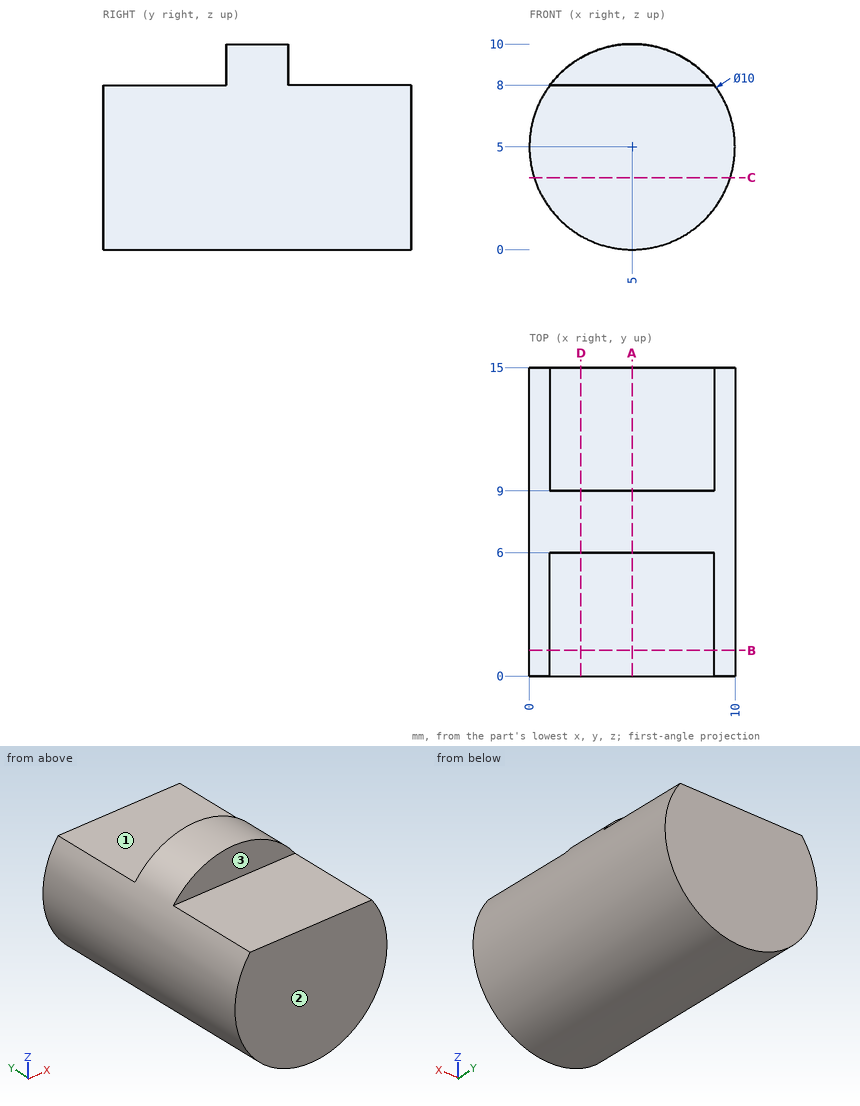
Source: three-view drawing plus pictorial views. Frame: mm from the lowest corner of the part. A direction names the side the tool comes from. Coordinates: 2 decimals unless noted, no trailing zeros. Loops run counter-clockwise (first coordinate to the right, second up) from the corner with the lowest first, then second, coordinate; pieces in that order, holes last. Notation, with made-up numbers: M 35,-23.5 L 64,-23.5 A34 ccw 64,8.5 Z; hole C 52,45 d8. An arc over 180 degrees is marked long. Use CSV: the item, a comma, the result in double quotes.
(1) Reachability of the marked faces 1, 2 and 3 from +Z, -Z, +X, -X, +Y, -Y: full face, straight path, thin tool, end or side. Return the list, or none.
Answers follow:
face 1,"+Z, +X, -X, +Y"
face 2,"+Z, -Z, +X, -X, -Y"
face 3,"+Z, +X, -X, -Y"
(2) Cut plane C-C on z = 3.5. Return loops of the section in (x, y), and give its area (3 significant figures).
Answers follow:
outline,"M 0.23,0 L 9.77,0 L 9.77,15 L 0.23,15 Z"
area,"143 mm²"
(3) Contact query for flat-ended pins moving along their axis: pin 1 (3 mm diameter, centred on x = 5.5, y = 2.5, fed in from +Z); pin 2 (1 mm diameter, centred on x = 6, z = 9, fed in from -Y); pin 3 (3 mm diameter, centred on x = 1, y = 5, fed in from -Z). Output: stop coordinate, or through.
Answers follow:
pin 1,"z = 8"
pin 2,"y = 6"
pin 3,"z = 0.67"
(4) Cut plane B-B on y = 1.25. Return loops of the section in (x, z).
Answers follow:
outline,"M 1,8 A5 ccw long 9,8 Z"
(5) Cut plane D-D on x = 2.5. Return loops of the section in (y, z), and give its area (3 significant figures).
Answers follow:
outline,"M 0,0.67 L 15,0.67 L 15,8 L 9,8 L 9,9.33 L 6,9.33 L 6,8 L 0,8 Z"
area,"114 mm²"
(6) Cut plane A-A on x = 5. Return loops of the section in (y, z), and give its area (3 significant figures).
Answers follow:
outline,"M 0,0 L 15,0 L 15,8 L 9,8 L 9,10 L 6,10 L 6,8 L 0,8 Z"
area,"126 mm²"
(7) Line query: line 1 (X direction, y = 10.25, z = 2); line 2 (Z direction, x = 5, y = 14); line 3 (X direction, y = 3, z = 6.5). Output: solid intervals per line, ascending. Write a range as [from, to].
Answers follow:
line 1,"[1, 9]"
line 2,"[0, 8]"
line 3,"[0.23, 9.77]"
